```python
from build123d import *

# Parameters (mm, degrees)
SKETCH1_W           = 60
SKETCH1_H           = 6.32
BOSS_EXTRUDE1_DEPTH = 10.64
SKETCH2_R           = 5
CUT_EXTRUDE1_DEPTH  = 64.974845056
SKETCH3_W           = 6.32
SKETCH3_H           = 21.28
BOSS_EXTRUDE2_DEPTH = 18.5
SKETCH4_W           = 6.32
SKETCH4_H           = 21.28
BOSS_EXTRUDE3_DEPTH = 18.5
SKETCH5_W           = 5
SKETCH5_H           = 21.28
BOSS_EXTRUDE6_DEPTH = 84.33
SKETCH6_W           = 5
SKETCH6_H           = 21.291954735
BOSS_EXTRUDE7_DEPTH = 84.33
SKETCH7_W           = 6.32
SKETCH7_H           = 21.291954735
BOSS_EXTRUDE8_DEPTH = 92
SKETCH9_R           = 5
CUT_EXTRUDE2_DEPTH  = 118.162904694
SKETCH10_R          = 2.22
CUT_EXTRUDE3_DEPTH  = 121.387443862
FILLET1_R           = 3
SKETCH13_R          = 2
CUT_EXTRUDE4_DEPTH  = 121.387443862


with BuildPart() as part:
    # Sketch1 → Boss-Extrude1 (new, symmetric)
    with BuildSketch(Plane(origin=(0, 0, 0), x_dir=(1, 0, 0), z_dir=(0, 1, 0))):
        with Locations((30, -3.16)):
            Rectangle(SKETCH1_W, SKETCH1_H)
    extrude(amount=BOSS_EXTRUDE1_DEPTH, both=True)

    # Sketch2 → Cut-Extrude1 (cut, through all)
    with BuildSketch(Plane(origin=(0, 10.64, 0), x_dir=(1, 0, 0), z_dir=(0, 1, 0))):
        with Locations((7.21, 1.25)):
            Circle(SKETCH2_R)
        with Locations((52.79, 1.25)):
            Circle(SKETCH2_R)
    extrude(amount=-CUT_EXTRUDE1_DEPTH, mode=Mode.SUBTRACT)

    # Sketch3 → Boss-Extrude2 (add)
    with BuildSketch(Plane(origin=(60, 0, 0), x_dir=(0, 0, -1), z_dir=(1, 0, 0))):
        with Locations((-3.16, 0)):
            Rectangle(SKETCH3_W, SKETCH3_H)
    extrude(amount=BOSS_EXTRUDE2_DEPTH)

    # Sketch4 → Boss-Extrude3 (add)
    with BuildSketch(Plane.ZY):
        with Locations((3.16, 0)):
            Rectangle(SKETCH4_W, SKETCH4_H)
    extrude(amount=BOSS_EXTRUDE3_DEPTH)

    # Sketch5 → Boss-Extrude6 (add)
    with BuildSketch(Plane(origin=(0, 0, 0), x_dir=(-1, 0, 0), z_dir=(0, 0, -1))):
        with Locations((16, 0)):
            Rectangle(SKETCH5_W, SKETCH5_H)
    extrude(amount=BOSS_EXTRUDE6_DEPTH)

    # Sketch6 → Boss-Extrude7 (add)
    with BuildSketch(Plane(origin=(0, 0, 0), x_dir=(-1, 0, 0), z_dir=(0, 0, -1))):
        with Locations((-76, -0.005977367)):
            Rectangle(SKETCH6_W, SKETCH6_H)
    extrude(amount=BOSS_EXTRUDE7_DEPTH)

    # Sketch7 → Boss-Extrude8 (add, through all)
    with BuildSketch(Plane.ZY.offset(-73.5)):
        with Locations((-81.17, -0.005977367)):
            Rectangle(SKETCH7_W, SKETCH7_H)
    extrude(amount=BOSS_EXTRUDE8_DEPTH)

    # Sketch9 → Cut-Extrude2 (cut, through all)
    with BuildSketch(Plane(origin=(0, 10.64, 0), x_dir=(1, 0, 0), z_dir=(0, 1, 0))):
        with Locations((7.21, 76.76)):
            Circle(SKETCH9_R)
        with Locations((52.79, 76.76)):
            Circle(SKETCH9_R)
    extrude(amount=-CUT_EXTRUDE2_DEPTH, mode=Mode.SUBTRACT)

    # Sketch10 → Cut-Extrude3 (cut, through all)
    with BuildSketch(Plane(origin=(0, 0, -84.33), x_dir=(-1, 0, 0), z_dir=(0, 0, -1))):
        with Locations((-62.631229183, 0.005)):
            Circle(SKETCH10_R)
        with Locations((2.631229183, 0.005)):
            Circle(SKETCH10_R)
    extrude(amount=-CUT_EXTRUDE3_DEPTH, mode=Mode.SUBTRACT)

    # Fillet1
    fillet1_edges = [part.edges().sort_by_distance(p)[0] for p in [
        (78.5, 0, 6.32),
        (-18.5, 0, 6.32),
        (-13.5, 0, 0),
        (-18.5, -0.005977367, -84.33),
        (73.5, 0, 0),
        (78.5, -0.005977367, -84.33),
        (-13.5, 0, -78.01),
        (73.5, -0.005977367, -78.01),
    ]]
    fillet(fillet1_edges, radius=FILLET1_R)

    # Sketch13 → Cut-Extrude4 (cut, through all)
    with BuildSketch(Plane(origin=(0, 0, -84.33), x_dir=(-1, 0, 0), z_dir=(0, 0, -1))):
        with Locations((-30, 0.005)):
            Circle(SKETCH13_R)
    extrude(amount=-CUT_EXTRUDE4_DEPTH, mode=Mode.SUBTRACT)


solid = part.part
```
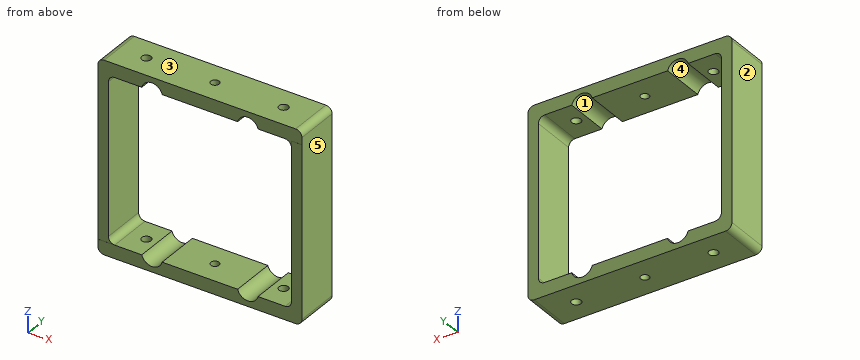
Source: CAD feature listing. Evaluate the final solid. Frame: model axes, mm. Face numbers are marked on the shaded views. A direction names the side the tool comes from. Give positions to 0.01 mm unless a question says otherwise; leave off trailing zeros. Order: outer loops, then holes, each group sorted by start corner. A loop starts at its lowest first (then second) coordinate and runs counter-clockwise, first axis right, second up. Notation, with made-up numbers: (2.25, -9) -> (18.25, -9) arc R11 ccw to (18.25, 11) -> close; hole circle Ø6 at (45.25, -16). An arc over 180 degrees is marked (long way). Use a Markdown table: item, result.
Q1. Pull-direction query (Z, two-part tool) for the marked faces 1, 2 and 3; classes: +Z half, -Z half, draft (parallel to the pull), parting line (faces both ways), or undercut.
A:
| item | result |
|---|---|
| face 1 | undercut |
| face 2 | draft |
| face 3 | +Z half |
Q2. Access query for the marked faces 4 and 5. Directions: +Z, -Z, +X, -X, +Y, -Y. A direction counts if a zero-diameter tool reaches every point of the face in a straight line with its end or side. Return the directions, or none.
A:
| item | result |
|---|---|
| face 4 | +Y, -Y |
| face 5 | +Z, -Z, +X, +Y, -Y |
Q3. Material intervals for line 1 (X direction, y = 7.75, z = -11); line 2 (Z direction, x = 60, y = -2.5); line 3 (Z direction, x = 7, y = 3.75), sorted ascending. Write a range as [from, to].
A:
| item | result |
|---|---|
| line 1 | [-18.5, -13.5], [73.5, 78.5] |
| line 2 | [-84.33, -78.01], [0, 6.32] |
| line 3 | [-84.33, -81.76], [3.75, 6.32] |
Q4. Section A-A (x = 30). Return the cut outline in (y, z) (3 decimals), and give its area (3 significant figures).
A:
| item | result |
|---|---|
| outline | (-10.652, -84.33) -> (-1.995, -84.33) -> (-1.995, -78.01) -> (-10.652, -78.01) -> close; (-10.64, 0) -> (-1.995, 0) -> (-1.995, 6.32) -> (-10.64, 6.32) -> close; (2.005, -84.33) -> (10.64, -84.33) -> (10.64, -78.01) -> (2.005, -78.01) -> close; (2.005, 0) -> (10.64, 0) -> (10.64, 6.32) -> (2.005, 6.32) -> close |
| area | 218 mm^2 |
Q5. Section C-C (y = 7). Return the cut outline in (x, z).
A:
| item | result |
|---|---|
| outline | (-18.5, -81.33) arc R3 ccw to (-15.5, -84.33) -> (75.5, -84.33) arc R3 ccw to (78.5, -81.33) -> (78.5, 3.32) arc R3 ccw to (75.5, 6.32) -> (-15.5, 6.32) arc R3 ccw to (-18.5, 3.32) -> close; hole (-13.5, -75.01) arc R3 ccw to (-10.5, -78.01) -> (2.37, -78.01) arc R5 ccw to (12.05, -78.01) -> (47.95, -78.01) arc R5 ccw to (57.63, -78.01) -> (70.5, -78.01) arc R3 ccw to (73.5, -75.01) -> (73.5, -3) arc R3 ccw to (70.5, 0) -> (57.63, 0) arc R5 ccw to (47.95, 0) -> (12.05, 0) arc R5 ccw to (2.37, 0) -> (-10.5, 0) arc R3 ccw to (-13.5, -3) -> close |
Q6. Section D-D (x = 50.5). Return the cut outline in (y, z).
A:
| item | result |
|---|---|
| outline | (-10.65, -84.33) -> (10.64, -84.33) -> (10.64, -81.2) -> (-10.65, -81.2) -> close; (-10.64, 3.19) -> (10.64, 3.19) -> (10.64, 6.32) -> (-10.64, 6.32) -> close |
Q7. Section B-B (z = -61). Return the cut outline in (x, y).
A:
| item | result |
|---|---|
| outline | (-18.5, -10.64) -> (-13.5, -10.64) -> (-13.5, 10.64) -> (-18.5, 10.64) -> close; (73.5, -10.65) -> (78.5, -10.65) -> (78.5, 10.64) -> (73.5, 10.64) -> close |
